Autodesk Inventor part; units mm, degrees
ref_plane "YZ Plane" through (0, 0, 0) normal (1, 0, 0) x (0, 1, 0)
ref_plane "XZ Plane" through (0, 0, 0) normal (0, 1, 0) x (-1, 0, 0)
ref_plane "XY Plane" through (0, 0, 0) normal (0, 0, 1) x (1, 0, 0)
sketch "Sketch1" plane through (0, 0, 0) normal (0, 1, 0) x (-1, 0, 0)
  point P0 (0, 0)
sketch "Sketch2" plane through (0, 0, 0) normal (0, 1, 0) x (-1, 0, 0)
  line L0 (105, 50) -> (-105, 50)
  line L1 (-105, 50) -> (-105, -50)
  line L2 (-105, -50) -> (105, -50)
  line L3 (105, -50) -> (105, 50)
  line L4 (105, 50) -> (-105, -50) construction
  line L5 (-105, 50) -> (105, -50) construction
  point P0 (0, 0)
  dimension "d0" = 210
  dimension "d1" = 100
extrude "Extrusion1" add sketch "Sketch2" along normal blind 3
sketch "Sketch3" plane through (0, 3, 0) normal (0, 1, 0) x (1, 0, 0)
  line L0 (-21, 0) -> (-18, 0)
  line L1 (-18, 0) -> (-18, 20)
  line L2 (-18, 20) -> (-21, 20)
  line L3 (-21, 20) -> (-21, 0)
  line L4 (-21, 0) -> (-18, 20) construction
  line L5 (-18, 0) -> (-21, 20) construction
  line L6 (105, 50) -> (-105, 50)
  line L7 (62, 20) -> (65, 20)
  line L8 (65, 20) -> (65, 0)
  line L9 (65, 0) -> (62, 0)
  line L10 (62, 0) -> (62, 20)
  line L11 (62, 20) -> (65, 0) construction
  line L12 (65, 20) -> (62, 0) construction
  line L13 (105, -50) -> (105, 50)
  line L14 (-21, -40) -> (-18, -40)
  line L15 (-18, -40) -> (-18, -20)
  line L16 (-18, -20) -> (-21, -20)
  line L17 (-21, -20) -> (-21, -40)
  line L18 (-21, -40) -> (-18, -20) construction
  line L19 (-18, -40) -> (-21, -20) construction
  line L20 (-105, -50) -> (105, -50)
  line L21 (62, -20) -> (65, -20)
  line L22 (65, -20) -> (65, -40)
  line L23 (65, -40) -> (62, -40)
  line L24 (62, -40) -> (62, -20)
  line L25 (62, -20) -> (65, -40) construction
  line L26 (65, -20) -> (62, -40) construction
  line L27 (-8, 24.65) -> (12, 24.65)
  line L28 (12, 24.65) -> (12, 21.65)
  line L29 (12, 21.65) -> (-8, 21.65)
  line L30 (-8, 21.65) -> (-8, 24.65)
  line L31 (-8, 24.65) -> (12, 21.65) construction
  line L32 (12, 24.65) -> (-8, 21.65) construction
  line L33 (32, 24.65) -> (52, 24.65)
  line L34 (52, 24.65) -> (52, 21.65)
  line L35 (52, 21.65) -> (32, 21.65)
  line L36 (32, 21.65) -> (32, 24.65)
  line L37 (32, 24.65) -> (52, 21.65) construction
  line L38 (52, 24.65) -> (32, 21.65) construction
  line L39 (-105, -50) -> (105, -50)
  line L40 (105, -50) -> (105, 50)
  line L41 (105, 50) -> (-105, 50)
  line L42 (-105, 50) -> (-105, -50)
  point P0 (0, 0)
  point P1 (-19.5, 10)
  point P2 (63.5, 10)
  point P3 (-19.5, -30)
  point P4 (63.5, -30)
  point P5 (2, 23.15)
  point P6 (42, 23.15)
  dimension "d4" = 3
  dimension "d5" = 20
  dimension "d6" = 30
  dimension "d7" = 3
  dimension "d8" = 20
  dimension "d9" = 30
  dimension "d10" = 80
  dimension "d11" = 40
  dimension "d14" = 20
  dimension "d15" = 10
  dimension "d16" = 20
  dimension "d17" = 3
  dimension "d18" = 10
  dimension "d19" = 20
  dimension "d20" = 3
  dimension "d21" = 10
extrude "Extrusion2" cut sketch "Sketch3" against normal through all contours L3 L2 L1 L0 | L7 L8 L9 L10
sketch "Sketch4" plane through (0, 3, 0) normal (0, 1, 0) x (1, 0, 0)
  point P0 (0, 0)
sketch "Sketch5" plane through (0, 3, 0) normal (0, 1, 0) x (1, 0, 0)
  line L0 (-21, 0) -> (-21, 20)
  line L1 (-18, 20) -> (-18, 0)
  line L2 (-21, 20) -> (-18, 20)
  line L3 (-18, 0) -> (-21, 0)
  line L4 (62, 0) -> (62, 20)
  line L5 (65, 0) -> (62, 0)
  line L6 (65, 20) -> (65, 0)
  line L7 (62, 20) -> (65, 20)
  point P0 (0, 0)
sketch "Sketch6" plane through (0, 3, 0) normal (0, 1, 0) x (1, 0, 0)
  line L0 (-21, 0) -> (-18, 0)
  line L1 (-18, 0) -> (-18, 20)
  line L2 (-18, 20) -> (-21, 20)
  line L3 (-21, 20) -> (-21, 0)
  line L4 (-21, 0) -> (-18, 20) construction
  line L5 (-18, 0) -> (-21, 20) construction
  line L6 (105, 50) -> (-105, 50)
  line L7 (62, 20) -> (65, 20)
  line L8 (65, 20) -> (65, 0)
  line L9 (65, 0) -> (62, 0)
  line L10 (62, 0) -> (62, 20)
  line L11 (62, 20) -> (65, 0) construction
  line L12 (65, 20) -> (62, 0) construction
  line L13 (105, -50) -> (105, 50)
  line L14 (-21, -40) -> (-18, -40)
  line L15 (-18, -40) -> (-18, -20)
  line L16 (-18, -20) -> (-21, -20)
  line L17 (-21, -20) -> (-21, -40)
  line L18 (-21, -40) -> (-18, -20) construction
  line L19 (-18, -40) -> (-21, -20) construction
  line L20 (-105, -50) -> (105, -50)
  line L21 (62, -20) -> (65, -20)
  line L22 (65, -20) -> (65, -40)
  line L23 (65, -40) -> (62, -40)
  line L24 (62, -40) -> (62, -20)
  line L25 (62, -20) -> (65, -40) construction
  line L26 (65, -20) -> (62, -40) construction
  line L27 (-8, 23) -> (12, 23)
  line L28 (12, 23) -> (12, 20)
  line L29 (12, 20) -> (-8, 20)
  line L30 (-8, 20) -> (-8, 23)
  line L31 (-8, 23) -> (12, 20) construction
  line L32 (12, 23) -> (-8, 20) construction
  line L33 (32, 23) -> (52, 23)
  line L34 (52, 23) -> (52, 20)
  line L35 (52, 20) -> (32, 20)
  line L36 (32, 20) -> (32, 23)
  line L37 (32, 23) -> (52, 20) construction
  line L38 (52, 23) -> (32, 20) construction
  line L39 (-105, -50) -> (105, -50)
  line L40 (105, -50) -> (105, 50)
  line L41 (105, 50) -> (-105, 50)
  line L42 (-105, 50) -> (-105, -50)
  point P0 (0, 0)
  point P1 (0, 0)
  point P2 (-19.5, 10)
  point P3 (63.5, 10)
  point P4 (-19.5, -30)
  point P5 (63.5, -30)
  point P6 (2, 21.5)
  point P7 (42, 21.5)
  dimension "d22" = 3
  dimension "d23" = 20
  dimension "d24" = 30
  dimension "d25" = 3
  dimension "d26" = 20
  dimension "d27" = 30
  dimension "d28" = 80
  dimension "d29" = 40
  dimension "d30" = 20
  dimension "d31" = 10
  dimension "d32" = 20
  dimension "d33" = 3
  dimension "d34" = 10
  dimension "d35" = 20
  dimension "d36" = 3
  dimension "d37" = 10
  dimension "d41" = 100
  dimension "d42" = 70
extrude "Extrusion3" cut sketch "Sketch6" against normal through all contours L17 L16 L15 L14 | L21 L22 L23 L24 | L27 L28 L29 L30 | L33 L34 L35 L36
sketch "Sketch7" plane through (0, 3, 0) normal (0, 1, 0) x (1, 0, 0)
  line L0 (-21, -40) -> (-21, -20)
  line L1 (-18, -20) -> (-18, -40)
  line L2 (-21, -20) -> (-18, -20)
  line L3 (-18, -40) -> (-21, -40)
  line L4 (62, -40) -> (62, -20)
  line L5 (65, -40) -> (62, -40)
  line L6 (65, -20) -> (65, -40)
  line L7 (62, -20) -> (65, -20)
  line L8 (-105, 50) -> (-105, -50)
  line L9 (-105, -50) -> (105, -50)
  line L10 (-95, -40) -> (-75, -40)
  line L11 (-75, -40) -> (-75, -37)
  line L12 (-75, -37) -> (-95, -37)
  line L13 (-95, -37) -> (-95, -40)
  line L14 (-55, -40) -> (-35, -40)
  line L15 (-35, -40) -> (-35, -37)
  line L16 (-35, -37) -> (-55, -37)
  line L17 (-55, -37) -> (-55, -40)
  line L18 (105, -50) -> (105, 50)
  line L19 (95, -40) -> (75, -40)
  line L20 (75, -40) -> (75, -37)
  line L21 (75, -37) -> (95, -37)
  line L22 (95, -37) -> (95, -40)
  line L23 (105, 50) -> (-105, 50)
  line L24 (-95, 40) -> (-92, 40)
  line L25 (-92, 40) -> (-92, 20)
  line L26 (-92, 20) -> (-95, 20)
  line L27 (-95, 20) -> (-95, 40)
  line L28 (-95, 0) -> (-92, 0)
  line L29 (-92, 0) -> (-92, -20)
  line L30 (-92, -20) -> (-95, -20)
  line L31 (-95, -20) -> (-95, 0)
  line L32 (95, 40) -> (92, 40)
  line L33 (92, 40) -> (92, 20)
  line L34 (92, 20) -> (95, 20)
  line L35 (95, 20) -> (95, 40)
  line L36 (95, -20) -> (92, -20)
  line L37 (92, -20) -> (92, 0)
  line L38 (92, 0) -> (95, 0)
  line L39 (95, 0) -> (95, -20)
  line L40 (-72, 103) -> (-62, 103)
  line L41 (-62, 103) -> (-62, 100)
  line L42 (-62, 100) -> (-72, 100)
  line L43 (-72, 100) -> (-72, 103)
  line L44 (-47, 103) -> (-37, 103)
  line L45 (-37, 103) -> (-37, 100)
  line L46 (-37, 100) -> (-47, 100)
  line L47 (-47, 100) -> (-47, 103)
  line L48 (-22, 103) -> (-12, 103)
  line L49 (-12, 103) -> (-12, 100)
  line L50 (-12, 100) -> (-22, 100)
  line L51 (-22, 100) -> (-22, 103)
  line L52 (3, 103) -> (13, 103)
  line L53 (13, 103) -> (13, 100)
  line L54 (13, 100) -> (3, 100)
  line L55 (3, 100) -> (3, 103)
  line L56 (28, 103) -> (38, 103)
  line L57 (38, 103) -> (38, 100)
  line L58 (38, 100) -> (28, 100)
  line L59 (28, 100) -> (28, 103)
  line L60 (53, 100) -> (63, 100)
  line L61 (63, 100) -> (63, 103)
  line L62 (63, 103) -> (53, 103)
  line L63 (53, 103) -> (53, 100)
  point P0 (0, 0)
  point P1 (-105, 48)
  point P2 (-105, -48)
  point P3 (-103, -50)
  point P4 (103, -50)
  point P5 (105, -48)
  point P6 (105, 48)
  point P7 (103, 50)
  point P8 (-103, 50)
  dimension "d43" = 10
  dimension "d44" = 10
  dimension "d45" = 20
  dimension "d46" = 3
  dimension "d47" = 20
  dimension "d48" = 3
  dimension "d49" = 20
  dimension "d50" = 10
  dimension "d51" = 10
  dimension "d52" = 20
  dimension "d53" = 3
  dimension "d54" = 10
  dimension "d55" = 10
  dimension "d56" = 10
  dimension "d57" = 10
  dimension "d58" = 3
  dimension "d59" = 20
  dimension "d60" = 3
  dimension "d61" = 20
  dimension "d62" = 20
  dimension "d63" = 3
  dimension "d64" = 20
  dimension "d65" = 20
  dimension "d66" = 10
  dimension "d67" = 3
  dimension "d68" = 20
  dimension "d69" = 10
  dimension "d70" = 3
  dimension "d71" = 15
  dimension "d72" = 10
  dimension "d73" = 10
  dimension "d74" = 10
  dimension "d75" = 15
  dimension "d76" = 15
  dimension "d77" = 15
  dimension "d78" = 10
  dimension "d79" = 15
  dimension "d82" = 140
extrude "Extrusion4" cut sketch "Sketch7" against normal through all contours L13 L12 L11 L10 | L17 L16 L15 L14 | L19 L20 L21 L22 | L24 L25 L26 L27 | L28 L29 L30 L31 | L35 L34 L33 L32 | L36 L37 L38 L39 | L40 L41 L42 L43 | L44 L45 L46 L47 | L48 L49 L50 L51 | L52 L53 L54 L55 | L56 L57 L58 L59 | L63 L62 L61 L60
sketch "Sketch8" plane through (0, 3, 0) normal (0, 1, 0) x (1, 0, 0)
  point P0 (0, 0)
sketch "Sketch9" plane through (0, 0, 0) normal (0, -1, 0) x (1, 0, 0)
  line L0 (105, -50) -> (-105, -50)
  line L1 (105, -50) -> (-105, -50)
  line L2 (-105, -50) -> (-105, -116)
  line L3 (-105, -116) -> (105, -116)
  line L4 (105, -116) -> (105, -50)
  point P0 (0, 0)
  dimension "d83" = 66
extrude "Extrusion5" add sketch "Sketch9" against normal blind 3
sketch "Sketch10" plane through (0, 3, 0) normal (0, 1, 0) x (1, 0, 0)
  line L0 (-21, -40) -> (-21, -20)
  line L1 (-18, -20) -> (-18, -40)
  line L2 (-21, -20) -> (-18, -20)
  line L3 (-18, -40) -> (-21, -40)
  line L4 (62, -40) -> (62, -20)
  line L5 (65, -40) -> (62, -40)
  line L6 (65, -20) -> (65, -40)
  line L7 (62, -20) -> (65, -20)
  line L8 (-105, 50) -> (-105, -50)
  line L9 (-105, -50) -> (105, -50)
  line L10 (-95, -40) -> (-75, -40)
  line L11 (-75, -40) -> (-75, -37)
  line L12 (-75, -37) -> (-95, -37)
  line L13 (-95, -37) -> (-95, -40)
  line L14 (-55, -40) -> (-35, -40)
  line L15 (-35, -40) -> (-35, -37)
  line L16 (-35, -37) -> (-55, -37)
  line L17 (-55, -37) -> (-55, -40)
  line L18 (105, -50) -> (105, 50)
  line L19 (95, -40) -> (75, -40)
  line L20 (75, -40) -> (75, -37)
  line L21 (75, -37) -> (95, -37)
  line L22 (95, -37) -> (95, -40)
  line L23 (105, 50) -> (-105, 50)
  line L24 (-95, 40) -> (-92, 40)
  line L25 (-92, 40) -> (-92, 20)
  line L26 (-92, 20) -> (-95, 20)
  line L27 (-95, 20) -> (-95, 40)
  line L28 (-95, 0) -> (-92, 0)
  line L29 (-92, 0) -> (-92, -20)
  line L30 (-92, -20) -> (-95, -20)
  line L31 (-95, -20) -> (-95, 0)
  line L32 (95, 40) -> (92, 40)
  line L33 (92, 40) -> (92, 20)
  line L34 (92, 20) -> (95, 20)
  line L35 (95, 20) -> (95, 40)
  line L36 (95, -20) -> (92, -20)
  line L37 (92, -20) -> (92, 0)
  line L38 (92, 0) -> (95, 0)
  line L39 (95, 0) -> (95, -20)
  line L40 (-72, 106) -> (-62, 106)
  line L41 (-62, 106) -> (-62, 103)
  line L42 (-62, 103) -> (-72, 103)
  line L43 (-72, 103) -> (-72, 106)
  line L44 (-47, 106) -> (-37, 106)
  line L45 (-37, 106) -> (-37, 103)
  line L46 (-37, 103) -> (-47, 103)
  line L47 (-47, 103) -> (-47, 106)
  line L48 (-22, 106) -> (-12, 106)
  line L49 (-12, 106) -> (-12, 103)
  line L50 (-12, 103) -> (-22, 103)
  line L51 (-22, 103) -> (-22, 106)
  line L52 (3, 106) -> (13, 106)
  line L53 (13, 106) -> (13, 103)
  line L54 (13, 103) -> (3, 103)
  line L55 (3, 103) -> (3, 106)
  line L56 (28, 106) -> (38, 106)
  line L57 (38, 106) -> (38, 103)
  line L58 (38, 103) -> (28, 103)
  line L59 (28, 103) -> (28, 106)
  line L60 (53, 103) -> (63, 103)
  line L61 (63, 103) -> (63, 106)
  line L62 (63, 106) -> (53, 106)
  line L63 (53, 106) -> (53, 103)
  line L64 (105, 116) -> (-105, 116)
  point P0 (0, 0)
  point P1 (0, 0)
  point P2 (-105, 48)
  point P3 (-105, -48)
  point P4 (-103, -50)
  point P5 (103, -50)
  point P6 (105, -48)
  point P7 (105, 48)
  point P8 (103, 50)
  point P9 (-103, 50)
  dimension "d86" = 10
  dimension "d87" = 10
  dimension "d88" = 20
  dimension "d89" = 3
  dimension "d90" = 20
  dimension "d91" = 3
  dimension "d92" = 20
  dimension "d93" = 10
  dimension "d94" = 10
  dimension "d95" = 20
  dimension "d96" = 3
  dimension "d97" = 10
  dimension "d98" = 10
  dimension "d99" = 10
  dimension "d100" = 10
  dimension "d101" = 3
  dimension "d102" = 20
  dimension "d103" = 3
  dimension "d104" = 20
  dimension "d105" = 20
  dimension "d106" = 3
  dimension "d107" = 20
  dimension "d108" = 20
  dimension "d109" = 10
  dimension "d110" = 3
  dimension "d111" = 20
  dimension "d112" = 10
  dimension "d113" = 3
  dimension "d114" = 15
  dimension "d115" = 10
  dimension "d116" = 10
  dimension "d117" = 10
  dimension "d118" = 15
  dimension "d119" = 15
  dimension "d120" = 15
  dimension "d121" = 10
  dimension "d122" = 15
  dimension "d126" = 10
  dimension "d127" = 3
extrude "Extrusion6" cut sketch "Sketch10" against normal through all contours L40 L41 L42 L43 | L44 L45 L46 L47 | L48 L49 L50 L51 | L52 L53 L54 L55 | L56 L57 L58 L59 | L63 L62 L61 L60
equation "\"d9\" = d6"
equation "\"d21\" = d18"
equation "\"d27\" = d24"
equation "\"d37\" = d34"
equation "\"d44\" = d43"
equation "\"d75\" = d71"
equation "\"d76\" = d75"
equation "\"d77\" = d76"
equation "\"d79\" = d76"
properties part number "base"
Design review of the part built by this model. Coordinates are the model's own, in mm. Give positions to 0.01 mm unless a question says otherwise; leave off trailing zeros. Write each loop counter-clockwise with the first axis right and the second up, starting at its lowest first coordinate (ties: lowest second). Pieces come first, ordered by that corner, then holes. Notation, with made-up numbers: (25, 85.25) -> (67, 85.25) arc R18 ccw to (67, 107.25) -> close; hole circle Ø3 at (87.25, 44). An arc over 180 degrees is marked (long way). Answer in a Markdown table with one row per item.
(1) Consider section B-B (z = -36). State the section outline as (x, y) points.
Results:
| item | result |
|---|---|
| outline | (-105, 0) -> (-95, 0) -> (-95, 3) -> (-105, 3) -> close; (-92, 0) -> (92, 0) -> (92, 3) -> (-92, 3) -> close; (95, 0) -> (105, 0) -> (105, 3) -> (95, 3) -> close |
(2) To check wall thickness, follow probe 1 along X at (y, z) = (2, 27); probe 2 along Z at (x, y) = (32.5, 2.15); probe 3 along X at (y, z) = (1.1, -33). State the ranges of each line that lie inside material, in increasing order.
Results:
| item | result |
|---|---|
| probe 1 | -105 to -21, -18 to 62, 65 to 105 |
| probe 2 | -116 to -106, -103 to -23, -20 to 50 |
| probe 3 | -105 to -95, -92 to 92, 95 to 105 |
(3) Consider section C-C (x = 9). State the section outline as (y, z) points, then the cut area to 3 significant figures.
Results:
| item | result |
|---|---|
| outline | (0, -116) -> (3, -116) -> (3, -106) -> (0, -106) -> close; (0, -103) -> (3, -103) -> (3, -23) -> (0, -23) -> close; (0, -20) -> (3, -20) -> (3, 50) -> (0, 50) -> close |
| area | 480 mm2 |
(4) Consider section D-D (y = 2.5). Count the separate pieces of the cut face and the enclosed holes in it, then the cut area to 3 significant figures.
Results:
| item | result |
|---|---|
| separate pieces | 1 |
| enclosed holes | 19 |
| area | 33,900 mm2 |
(5) Consider section A-A (x = 56). State the section outline as (y, z) points.
Results:
| item | result |
|---|---|
| outline | (0, -116) -> (3, -116) -> (3, -106) -> (0, -106) -> close; (0, -103) -> (3, -103) -> (3, 50) -> (0, 50) -> close |
